```python
from build123d import *

# Parameters (mm, degrees)
F2_DEPTH = 2
F3_T     = 7
F4_R     = 4
F6_DEPTH = 11
F7_R     = 2.99999


# Not quite as in the source:
# - a fillet or chamfer is up to 0.001 mm smaller than in the source, because OpenCascade refuses the exact size
# - a shell that OpenCascade refuses in one call is made with other operations: the cavity is built on its own and cut out


with BuildPart() as f2:
    # F1 (on Top) → F2 (new body)
    with BuildSketch(Plane.XY):
        with BuildLine():
            ThreePointArc((-21.6449442268, 42.3033521048), (-25.6894079684, 40.4398561051), (-26.6437804137, 36.0902035288))
            Line((-26.6437804137, 36.0902035288), (-18.5483854863, 3.7846369171))
            ThreePointArc((-18.5483854863, 3.7846369171), (-16.7743151531, 1.0581212972), (-13.6983450146, 0))
            Line((-13.6983450146, 0), (12.2689166074, 0))
            ThreePointArc((12.2689166074, 0), (16.5100865033, 1.4311152002), (19.017084198, 5.1392920247))
            Line((19.017084198, 5.1392920247), (27.1577014469, 34.6625972473))
            ThreePointArc((27.1577014469, 34.6625972473), (26.3599974025, 38.9615518502), (22.4863774545, 40.9894598656))
            Line((22.4863774545, 40.9894598656), (-21.6449442268, 42.3033521048))
        make_face()
    extrude(amount=F2_DEPTH)

    # F3: shell of thickness 7, made by hand


with BuildPart() as f3_core1:
    # F3_t2: copy of F2
    add(f2.part)

    # the walls: a layer under each face that stays
    f3_faces = [f3_core1.faces().sort_by_distance(p)[0] for p in [
        (0.4207166138, 41.6464059852, 1),
        (-22.59608295, 19.937420223, 1),
        (-0.7147142036, 0, 1),
        (23.0873928224, 19.900944636, 1),
    ]]
    thicken(f3_faces, amount=-F3_T, mode=Mode.SUBTRACT)


with BuildPart() as f2_1:
    add(f2.part)

    # what is left inside the walls is the cavity
    f3_cavity = [f3_core1.part.solids().sort_by_distance(p)[0] for p in [
        (0.260689, 16.409264, 0.07),
    ]]
    add(f3_cavity, mode=Mode.SUBTRACT)

    # F4
    f4_edges = [f2_1.edges().sort_by_distance(p)[0] for p in [
        (19.732614, 34.068344, 1),
        (-19.211236, 35.227793, 1),
        (-12.137683, 7, 1),
        (12.268917, 7, 1),
    ]]
    fillet(f4_edges, radius=F4_R)

    # F5 (on face) → F6 (join)
    with BuildSketch(Plane.XY):
        Polygon((-23.3953947844, 35.4691530951), (-26.3054190674, 34.7399352453), (-24.8469833679, 28.9198866794), (-21.9369590849, 29.6491045291), align=None)
        Polygon((25.3943994744, 28.2676887604), (26.9892920247, 34.0518324094), (24.0972202001, 34.8492786846), (22.5023276498, 29.0651350355), align=None)
        Polygon((-19.3778494948, 7.0947045569), (-16.4678252118, 7.8239224066), (-17.9262609113, 13.6439709726), (-20.8362851943, 12.9147531229), align=None)
        Polygon((18.249280849, 13.6407519713), (16.6543882988, 7.8566083223), (19.5464601233, 7.0591620471), (21.1413526736, 12.8433056962), align=None)
    extrude(amount=-F6_DEPTH)

    # F7 (radius 3 in the source; OpenCascade refuses exactly that, so slightly less here)
    f7_edges = [f2_1.edges().sort_by_distance(p)[0] for p in [
        (25.543256, 34.450556, -11),
        (23.948364, 28.666412, -11),
        (19.695317, 13.242029, -11),
        (18.100424, 7.457885, -11),
        (-17.922837, 7.459313, -11),
        (-19.381273, 13.279362, -11),
        (-23.391971, 29.284496, -11),
        (-24.850407, 35.104544, -11),
    ]]
    fillet(f7_edges, radius=F7_R)


solid = f2_1.part
```
The model under review builds one solid part; all positions refer to its coordinate system, in mm. A direction names the side the tool comes from. Round coordinates to 2 decimals unless told otherwise and drop trailing zeros. Write each loop counter-clockwise with the first axis right and the second up, starting at its lowest first coordinate (ties: lowest second). Pieces come first, ordered by that corner, then holes. Notation, with made-up numbers: (0, 56) - (37, 56) arc R11 ccw to (37, 68) - close; hole circle Ø5 at (32, 35). An arc over 180 degrees is marked (long way). One line per question, with ' | ' between items.
Item 1: To check wall thickness, follow probe 1 along Z at (x, y) = (-21, 18.5); probe 2 along X at (y, z) = (9.5, 0.75); probe 3 along X at (y, z) = (33, 0.75). State the ranges of each line that lie inside material, in increasing order.
Resolved:
probe 1: z = 0 to 2 | probe 2: x = -19.98 to -12.72, 12.93 to 20.22 | probe 3: x = -25.87 to -17.55, 17.4 to 26.7
Item 2: Add section C-C, the plane z = -4.5. Give the boundary of the cut face in (x, y), then the cut area to 3 significant figures.
Resolved:
outline: (-26.31, 34.74) - (-24.85, 28.92) - (-21.94, 29.65) - (-23.4, 35.47) - close; (-20.84, 12.91) - (-19.38, 7.09) - (-16.47, 7.82) - (-17.93, 13.64) - close; (16.65, 7.86) - (19.55, 7.06) - (21.14, 12.84) - (18.25, 13.64) - close; (22.5, 29.07) - (25.39, 28.27) - (26.99, 34.05) - (24.1, 34.85) - close | area: 72.0 mm2
Item 3: The part is to be moulded in two halves that separate along X. For faces 1 (the face through (-16.811, 1.087, 0.986)), 2 (the face through (-11.51, 7.87, 1.01)), 3 (the face through (18.35, 8.28, -10.1)), 4 (the face through (19.45, 12.42, -10.1)), say which applies: pulls with the +X half, pulls with the -X half, needs draft (parallel to the pull), parting line crosses it, or undercut.
Resolved:
face 1: pulls with the -X half | face 2: undercut | face 3: undercut | face 4: pulls with the +X half
Item 4: For P1, Ø2, axis at x = 3, z = 1, coming from the +Y side; P2, Ø4, axis at x = -10, y = 10, coming from the -Z side; P3, Ø5, axis at y = 20.5, z = -1, coming from the -X side; P4, Ø6, axis at y = 34, z = -2.5, coming from the +X side, all flat-tipped, find the tip position at first contact; note any pin that passes through.
Resolved:
P1: stops at y = 41.6 | P2: passes through | P3: stops at x = -23.31 | P4: stops at x = 27.33
Item 5: Add section B-B, the plane y = 27. Give the boundary of the cut face in (x, z).
Resolved:
outline: (-24.37, 0) - (-17.15, 0) - (-17.15, 2) - (-24.37, 2) - close; (17.78, 0) - (25.04, 0) - (25.04, 2) - (17.78, 2) - close
Item 6: Add section A-A, the plane z = 1.25. Give the boundary of the cut face in (x, y).
Resolved:
outline: (-26.64, 36.09) - (-18.55, 3.78) arc R5 ccw to (-13.7, 0) - (12.27, 0) arc R7 ccw to (19.02, 5.14) - (27.16, 34.66) arc R5 ccw to (22.49, 40.99) - (-21.64, 42.3) arc R5 ccw to start; hole (-17.93, 30.1) - (-12.9, 10.03) arc R4 ccw to (-9.02, 7) - (9.22, 7) arc R4 ccw to (13.08, 9.94) - (18.38, 29.16) arc R4 ccw to (14.64, 34.22) - (-13.93, 35.07) arc R4 ccw to start
Item 7: Add section D-D, the plane x = 8. Give the boundary of the cut face in (y, z).
Resolved:
outline: (0, 0) - (7, 0) - (7, 2) - (0, 2) - close; (34.42, 0) - (41.42, 0) - (41.42, 2) - (34.42, 2) - close
Item 8: For faces 5 (the face through (-19.361, 13.284, -3.944)), 6 (the face through (11.62, 7.8, 1.01)), 7 (the face through (19.716, 13.236, -3.944)), list the 3-axis set-ups (+Z, -Z, +X, -X, +Y, -Y) from which the entire face can be reached by the end or side of a thin tool; tool diameter is ignored.
Resolved:
face 5: -Z, -X, +Y | face 6: +Z, -Z | face 7: -Z, +X, +Y
